Answer from the drawing. Dimensions are ordinates in mm from the lowest x, y and z of the part. Coordinates: 2 decimals unless noted, no trailing zeros. Order: outer loops, then holes, each group sorted by start corner. A loop starts at its lowest first (then second) coordinate and runs counter-clockwise, first axis right, second up. Notation, with made-up numbers: (45.5, 51) - (72.5, 51) arc R20 cw to (72.5, 80) - close; hole circle Ø9 at (-20, 89). An arc over 180 degrees is marked (long way). Use a Markdown table: item, result. Add a question column.
Item 1: Flat-ended cylindrical pins translate along their axes: P1, Ø3, axis at x = 88.5, z = 5.5, coming from the -Y side; P2, Ø5, axis at x = 229, y = 269, coming from the +Z side. Find the tip coordinate at first contact, or state that the pin passes through.
Item 2: The part is cut by section A-A, the plane z = 5.25. State how many separate pieces and enclosed holes the cut face has, then the cut area to 3 significant figures.
Item 3: The part is cut by section B-B, the plane y = 139. Give the vertices of the cut face in (x, z), then the cut area to 3 significant figures.
Item 4: Find the intervals of material crossed by line 1 along X through (y, z) = (179, 4.25); line 2 along Y through (x, z) = (229, 2), in increasing order.
Item 5: The part is cut by section C-C, the plane x = 170. Give the vertices of the cut face in (y, z), then the cut area to 3 significant figures.
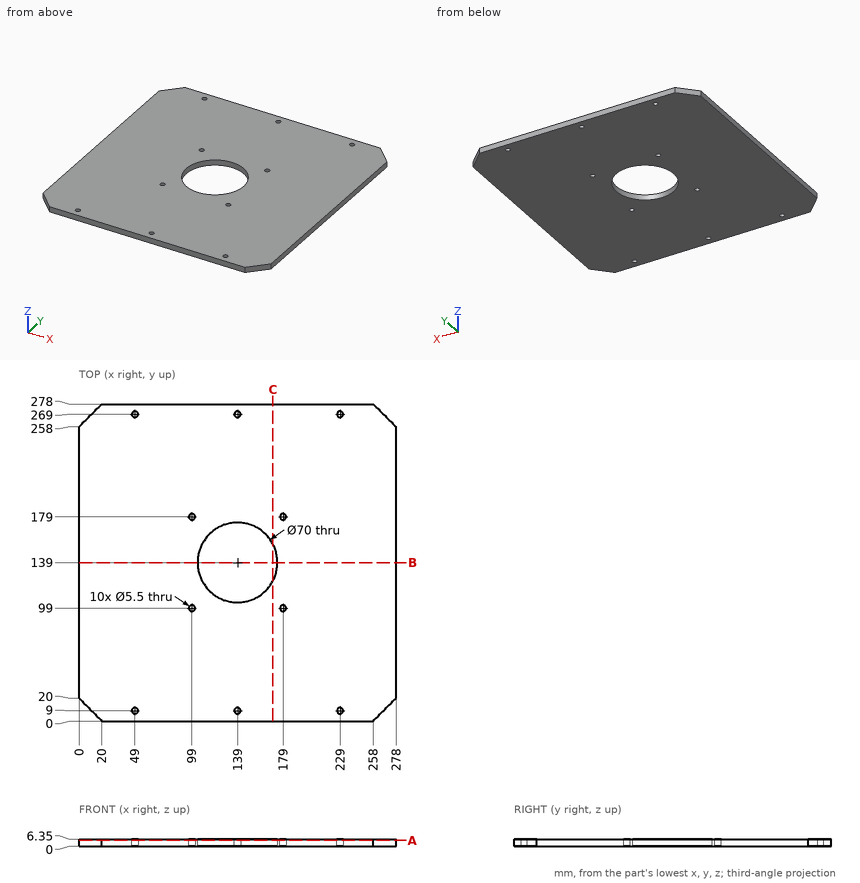
Solution:
| question | item | result |
|---|---|---|
| 1 | P1 | stops at y = 0 |
| 1 | P2 | passes through |
| 2 | separate pieces | 1 |
| 2 | enclosed holes | 11 |
| 2 | area | 72,400 mm2 |
| 3 | outline | (0, 0) - (104, 0) - (104, 6.35) - (0, 6.35) - close; (174, 0) - (278, 0) - (278, 6.35) - (174, 6.35) - close |
| 3 | area | 1,320 mm2 |
| 4 | line 1 | x = 0 to 96.25, 101.75 to 176.25, 181.75 to 278 |
| 4 | line 2 | y = 0 to 6.25, 11.75 to 266.25, 271.75 to 278 |
| 5 | outline | (0, 0) - (122.75, 0) - (122.75, 6.35) - (0, 6.35) - close; (155.25, 0) - (278, 0) - (278, 6.35) - (155.25, 6.35) - close |
| 5 | area | 1,560 mm2 |
